```python
from build123d import *

# Parameters (mm, degrees)
SKETCH1_R               = 2.4384
SKETCH1_R_2             = 1.397
BOSS_EXTRUDE1_DEPTH     = 25.49906
CROQUIS1_R              = 1.8161
SALIENTE_EXTRUIR1_DEPTH = 11
CROQUIS2_R              = 1.8161
SALIENTE_EXTRUIR2_DEPTH = 8


with BuildPart() as part:
    # Sketch1 → Boss-Extrude1 (new body)
    with BuildSketch(Plane.XY):
        Circle(SKETCH1_R)
        Circle(SKETCH1_R_2, mode=Mode.SUBTRACT)
    extrude(amount=BOSS_EXTRUDE1_DEPTH)

    # Croquis1 → Saliente-Extruir1 (add)
    with BuildSketch(Plane.XY.offset(25.49906)):
        Circle(CROQUIS1_R)
    extrude(amount=SALIENTE_EXTRUIR1_DEPTH)

    # Croquis2 → Saliente-Extruir2 (add, symmetric)
    with BuildSketch(Plane(origin=(0, 0, 0), x_dir=(-1, 0, 0), z_dir=(0, 0, -1))):
        with Locations(Location((0, 0, 0), (0, 0, 180))):
            Circle(CROQUIS2_R)
    extrude(amount=SALIENTE_EXTRUIR2_DEPTH, both=True)


solid = part.part
```
For this review, take the finished solid that the model builds, in its own axes (mm). A direction names the side the tool comes from. Give positions to 0.01 mm unless a question says otherwise; leave off trailing zeros. Order: outer loops, then holes, each group sorted by start corner. A loop starts at its lowest first (then second) coordinate and runs counter-clockwise, first axis right, second up.
1) Wall thickness on line 1 (Z direction, x = 1.1, y = -0.75); line 2 (Y direction, x = 0, z = 20.25); line 3 (Z direction, x = 1.7, y = 1.6): over which ranges is each line inside the solid? List them lowest first.
2) The part is to be moulded in two halves that separate along X. For faces 6 (the face through (0, 2, 25.499)), 7 (the face through (2.326, 0.732, 12.571)), 8 (the face through (-1.11, -0.85, 16.63)), say which applies: released by +X, released by -X, zero draft, split by the parting line, or undercut.
3) Take a section at C-C (z = 8.5). Give the boundary of the cut face in (x, y), then the cut area to 3 significant figures.
4) For faces 1 (the face through (1.73, 0.55, 30.92)), 2 (the face through (1.73, -0.55, -4.06)), 3 (the face through (0, 0, 36.499)), 4 (the face through (0, 0, 8)), 5 (the face through (0, 0, -8)), list the 3-axis set-ups (+Z, -Z, +X, -X, +Y, -Y) from which the entire face can be reached by the end or side of a thin tool; tool diameter is ignored.
5) Take a section at A-A (y = 0). Give the boundary of the cut face in (x, z), then the cut area to 3 significant figures.
Derived:
1. line 1: z = -8 to 8, 25.5 to 36.5
1. line 2: y = -2.44 to -1.4, 1.4 to 2.44
1. line 3: z = 0 to 25.5
2. face 6: zero draft
2. face 7: split by the parting line
2. face 8: undercut
3. outline: circle Ø4.88 at (0, 0); hole circle Ø2.79 at (0, 0)
3. area: 12.5 mm2
4. face 1: +Z
4. face 2: -Z
4. face 3: +Z, +X, -X, +Y, -Y
4. face 4: none
4. face 5: -Z, +X, -X, +Y, -Y
5. outline: (-2.44, 0) - (-1.82, 0) - (-1.82, -8) - (1.82, -8) - (1.82, 0) - (2.44, 0) - (2.44, 25.5) - (1.82, 25.5) - (1.82, 36.5) - (-1.82, 36.5) - (-1.82, 25.5) - (-2.44, 25.5) - close; hole (-1.4, 8) - (1.4, 8) - (1.4, 25.5) - (-1.4, 25.5) - close
5. area: 144 mm2
